Autodesk Inventor part; units mm, degrees
ref_plane "YZ Plane" through (0, 0, 0) normal (1, 0, 0) x (0, 1, 0)
ref_plane "XZ Plane" through (0, 0, 0) normal (0, 1, 0) x (-1, 0, 0)
ref_plane "XY Plane" through (0, 0, 0) normal (0, 0, 1) x (1, 0, 0)
sketch "Boceto1" plane through (0, 0, 0) normal (1, 0, 0) x (0, 1, 0)
  circle A0 centre (0, 0) radius 28.5
  dimension "d0" = 57
extrude "cuerpo" add sketch "Boceto1" along normal blind 40
sketch "Boceto2" plane through (40, 0, 0) normal (1, 0, 0) x (0, 0, -1)
  line L0 (-24.5, 28.5) -> (24.5, 28.5)
  line L1 (28.5, 24.5) -> (28.5, -24.5)
  line L2 (24.5, -28.5) -> (-24.5, -28.5)
  line L3 (-28.5, -24.5) -> (-28.5, 24.5)
  line L4 (-28.5, 28.5) -> (28.5, -28.5) construction
  line L5 (28.5, 28.5) -> (-28.5, -28.5) construction
  arc A0 (28.5, 24.5) -> (24.5, 28.5) centre (24.5, 24.5) ccw
  arc A1 (-24.5, 28.5) -> (-28.5, 24.5) centre (-24.5, 24.5) ccw
  arc A2 (-28.5, -24.5) -> (-24.5, -28.5) centre (-24.5, -24.5) ccw
  arc A3 (24.5, -28.5) -> (28.5, -24.5) centre (24.5, -24.5) ccw
  point P0 (0, 0)
  dimension "d3" = 57
  dimension "d4" = 57
  dimension "d16" = 4
extrude "cara" add sketch "Boceto2" along normal blind 5
sketch "Boceto3" plane through (45, 0, 0) normal (1, 0, 0) x (0, 0, -1)
  circle A0 centre (0, 0) radius 19
  dimension "d7" = 38
extrude "Extrusión3" add sketch "Boceto3" along normal blind 1.5
sketch "Boceto4" plane through (46.5, 0, 0) normal (1, 0, 0) x (0, 0, -1)
  circle A0 centre (0, 0) radius 4
  dimension "d10" = 8
extrude "Extrusión4" cut sketch "Boceto4" against normal blind 1.5
sketch "Boceto5" plane through (45, 0, 0) normal (1, 0, 0) x (0, 0, -1)
  circle A0 centre (0, 0) radius 3
  dimension "d13" = 6
extrude "Extrusión5" add sketch "Boceto5" along normal blind 20
sketch "Boceto6" plane through (45, 0, 0) normal (1, 0, 0) x (0, 0, -1)
  line L0 (24.5, 28.5) -> (-24.5, 28.5)
  line L1 (-28.5, 24.5) -> (-28.5, -24.5)
  line L2 (-28.5, 0) -> (28.2081, 0)
  line L3 (0, 28.5) -> (0, -28.5)
  line L4 (-24.5, -28.5) -> (24.5, -28.5)
  line L5 (-24.5, -28.5) -> (-23.5, -28.5)
  line L6 (0, -28.5) -> (-24.5, -28.5)
  line L7 (-23.5, -28.5) -> (-23.5, -23.5)
  circle A0 centre (-23.5, -23.5) radius 3
  circle A1 centre (23.5, -23.5) radius 3
  circle A2 centre (-23.5, 23.5) radius 3
  circle A3 centre (23.5, 23.5) radius 3
  point P0 (0, 0)
  dimension "d22" = 1
  dimension "d23" = 5
  dimension "d24" = 6
extrude "Extrusión6" cut sketch "Boceto6" against normal up to surface (5 mm away)
Geometry: final body of the model. Coordinates: model frame, mm. A direction names the side the tool comes from. Round coordinates to 2 decimals unless told otherwise and drop trailing zeros. Order: outer loops, then holes, each group sorted by start corner. A loop starts at its lowest first (then second) coordinate and runs counter-clockwise, first axis right, second up. Notation, with made-up numbers: (-27, 33) -> (-20, 33) arc R8 ccw to (-20, 39) -> close; hole circle Ø6 at (76, 70.25). An arc over 180 degrees is marked (long way). Write each question's results on one line, items separated by ' | '.
Q1. Access query for faces 1 (the face through (40, 21, -21)), 2 (the face through (45, 3, -1)), 3 (the face through (40, -20.5, 21.7)), 4 (the face through (40, 21.7, 20.6)). Directions: +Z, -Z, +X, -X, +Y, -Y. A direction counts if a zero-diameter tool reaches every point of the face in a straight line with its end or side. Return the directions, or none.
Response values:
face 1: -Z, -X, +Y | face 2: +X | face 3: +Z, -X, -Y | face 4: +Z, -X, +Y
Q2. Section query D-D (x = 59). Output: boundary loops of the cut face in (y, z), and give its area (3 significant figures).
Response values:
outline: circle Ø6 at (0, 0) | area: 28.3 mm²
Q3. Pin query (flat end, axial travel): pin 1 Ø10 at (x, z) = (33.5, -8.5) entering from -Y; pin 2 Ø8 at (x, y) = (34.5, -3.5) entering from -Z; pin 3 Ø5 at (x, z) = (51.5, 5) entering from -Y; pin 4 Ø8 at (y, z) = (23.5, 23.5) entering from -X. Return the tip coordinate at first contact, or that it passes through.
Response values:
pin 1: y = -28.28 | pin 2: z = -28.5 | pin 3: y = -1.66 | pin 4: x = 40
Q4. Section query C-C (z = 6). Output: boundary loops of the cut face in (x, y).
Response values:
outline: (0, -27.86) -> (40, -27.86) -> (40, -28.5) -> (45, -28.5) -> (45, -18.03) -> (46.5, -18.03) -> (46.5, 18.03) -> (45, 18.03) -> (45, 28.5) -> (40, 28.5) -> (40, 27.86) -> (0, 27.86) -> close
Q5. Pull-direction query (Z, two-part tool) for faces 5 (the face through (40, -21.6, -20.5)), 6 (the face through (45.76, -3.905, 0.867)), 7 (the face through (45.74, 16.856, -8.767)); classes: released by +Z, released by -Z, zero draft, split by the parting line, or undercut.
Response values:
face 5: zero draft | face 6: undercut | face 7: split by the parting line
Q6. Section query A-A (y = -23.5). Output: boundary loops of the cut face in (x, z).
Response values:
outline: (0, -16.12) -> (40, -16.12) -> (40, -20.5) -> (45, -20.5) -> (45, 20.5) -> (40, 20.5) -> (40, 16.12) -> (0, 16.12) -> close; (40, -28.5) -> (45, -28.5) -> (45, -26.5) -> (40, -26.5) -> close; (40, 26.5) -> (45, 26.5) -> (45, 28.5) -> (40, 28.5) -> close
Q7. Ray query, line 1 along Y through (x, z) = (45.65, 0); line 2 along Y through (x, z) = (41.9, -23.5); line 3 along Y through (x, z) = (53.5, 0). Return the intervals inside material, ascending.
Response values:
line 1: -19 to -4, -3 to 3, 4 to 19 | line 2: -28.5 to -26.5, -20.5 to 20.5, 26.5 to 28.5 | line 3: -3 to 3
